Here's how the part is built. I have some questions about the finished solid (model axes, mm). A direction names the side the tool comes from. Round coordinates to 2 decimals unless told otherwise and drop trailing zeros. Order: outer loops, then holes, each group sorted by start corner. A loop starts at its lowest first (then second) coordinate and runs counter-clockwise, first axis right, second up. Notation, with made-up numbers: (55.5, -3.75) -> (99.5, -3.75) arc R21 cw to (99.5, 30.25) -> close; hole circle Ø1 at (-17, 41.5). An arc over 180 degrees is marked (long way). Answer in a Markdown table with one row per item.
```python
from build123d import *

# Parameters (mm, degrees)
F1_DEPTH = 10
F2_R     = 1.5
F4_R     = 5
F3_R     = 3.1
F5_DEPTH = 2.5


with BuildPart() as f1:
    # F0 (on Top) → F1 (new body)
    with BuildSketch(Plane.XY):
        Polygon((0, 1), (-5.773, 1), (-5.773, -1), (0, -1), (5.773, -1), (5.773, 1), align=None)
        Polygon((-5.773, 1), (-5.773, 2.3094010768), (-9.773, 4.6188021535), (-13.773, 2.3094010768), (-13.773, -2.3094010768), (-9.773, -4.6188021535), (-5.773, -2.3094010768), (-5.773, -1), align=None)
        Polygon((-9.773, 3.2620290209), (-6.948, 1.6310145105), (-6.948, -1.6310145105), (-9.773, -3.2620290209), (-12.598, -1.6310145105), (-12.598, 1.6310145105), align=None, mode=Mode.SUBTRACT)
        Polygon((5.773, 2.3094010768), (5.773, 1), (5.773, -1), (5.773, -2.3094010768), (9.773, -4.6188021535), (13.773, -2.3094010768), (13.773, 2.3094010768), (9.773, 4.6188021535), align=None)
        Polygon((6.948, 1.6310145105), (9.773, 3.2620290209), (12.598, 1.6310145105), (12.598, -1.6310145105), (9.773, -3.2620290209), (6.948, -1.6310145105), align=None, mode=Mode.SUBTRACT)
    extrude(amount=F1_DEPTH)

    # F2
    f2_edges = [f1.edges().sort_by_distance(p)[0] for p in [
        (-9.773, -4.618802, 5),
        (-13.773, -2.309401, 5),
        (-13.773, 2.309401, 5),
        (-9.773, 4.618802, 5),
        (-5.773, 2.309401, 5),
        (-5.773, -2.309401, 5),
        (5.773, 2.309401, 5),
        (9.773, 4.618802, 5),
        (13.773, 2.309401, 5),
        (13.773, -2.309401, 5),
        (9.773, -4.618802, 5),
        (5.773, -2.309401, 5),
    ]]
    fillet(f2_edges, radius=F2_R)

    # F4
    f4_edges = [f1.edges().sort_by_distance(p)[0] for p in [
        (-5.773, -1, 5),
        (-5.773, 1, 5),
        (5.773, 1, 5),
        (5.773, -1, 5),
    ]]
    fillet(f4_edges, radius=F4_R)

    # F3 (on face) → F5 (cut, symmetric)
    with BuildSketch(Plane.XZ.offset(1)):
        with Locations((0, 5)):
            Circle(F3_R)
    extrude(amount=F5_DEPTH, both=True, mode=Mode.SUBTRACT)


solid = f1.part
```
1. Suppose I cut it at A-A on y = 0.5. Write out the boundary of the cut face in (x, z), then the cut area to 3 significant figures.
Numbers:
| item | result |
|---|---|
| outline | (-13.77, 0) -> (-12.6, 0) -> (-12.6, 10) -> (-13.77, 10) -> close; (-6.95, 0) -> (6.95, 0) -> (6.95, 10) -> (-6.95, 10) -> close; (12.6, 0) -> (13.77, 0) -> (13.77, 10) -> (12.6, 10) -> close; hole circle Ø6.2 at (0, 5) |
| area | 132 mm2 |
2. Suppose I cut it at C-C on z = 5. State how many separate pieces and enclosed holes the cut face has, then the cut area to 3 significant figures.
Numbers:
| item | result |
|---|---|
| separate pieces | 2 |
| enclosed holes | 2 |
| area | 69.4 mm2 |
3. We'd pull the mould along X, two halves only. Please class faces 1 (the face through (-11.79, -3.454, 4.93)), 2 (the face through (6.948, 0, 5)), 3 (the face through (7.756, -3.454, 4.93)), 4 (the face through (13.57, -2.2, 5.07)): released by +X, released by -X, zero draft, split by the parting line, or undercut.
Numbers:
| item | result |
|---|---|
| face 1 | released by -X |
| face 2 | undercut |
| face 3 | undercut |
| face 4 | released by +X |
4. Please list where these lines run through material, in increasing order: line 1 along X through (y, z) = (0.6, 5); line 2 along X through (y, z) = (0, 0.75); line 3 along X through (y, z) = (-2.75, 8.5).
Numbers:
| item | result |
|---|---|
| line 1 | x = -13.77 to -12.6, -6.95 to -3.1, 3.1 to 6.95, 12.6 to 13.77 |
| line 2 | x = -13.77 to -12.6, -6.95 to 6.95, 12.6 to 13.77 |
| line 3 | x = -13.01 to -10.66, -8.89 to -6.54, 6.54 to 8.89, 10.66 to 13.01 |
5. For pin 1 Ø1 at (x, z) = (-5.5, 5) entering from +Y; pin 2 Ø1 at (x, z) = (0.5, 9) entering from -Y; pin 3 Ø1 at (x, z) = (0, 8) entering from +Y, each with a flat end and sliding along its axis, tell me the tip position at first contact or that it passes through.
Numbers:
| item | result |
|---|---|
| pin 1 | stops at y = 2.3 |
| pin 2 | stops at y = -1 |
| pin 3 | stops at y = 1 |
6. Suppose I cut it at B-B on x = 0. Write out the boundary of the cut face in (y, z).
Numbers:
| item | result |
|---|---|
| outline | (-1, 0) -> (1, 0) -> (1, 1.9) -> (-1, 1.9) -> close; (-1, 8.1) -> (1, 8.1) -> (1, 10) -> (-1, 10) -> close |
7. For faces 5 (the face through (-13.58, 2.18, 5.07)), 6 (the face through (-6.948, 0, 5)), 7 (the face through (-7.756, 3.454, 4.93)), which set-ups out of +Z, -Z, +X, -X, +Y, -Y let a thin tool reach every point of the face, with its end or its side?
Numbers:
| item | result |
|---|---|
| face 5 | +Z, -Z, -X, +Y |
| face 6 | +Z, -Z |
| face 7 | +Z, -Z, +Y |
